Autodesk Inventor part; units mm, degrees
ref_plane "YZ Plane" through (0, 0, 0) normal (1, 0, 0) x (0, 1, 0)
ref_plane "XZ Plane" through (0, 0, 0) normal (0, 1, 0) x (-1, 0, 0)
ref_plane "XY Plane" through (0, 0, 0) normal (0, 0, 1) x (1, 0, 0)
sketch "Sketch1" plane through (0, 0, 0) normal (0, 1, 0) x (-1, 0, 0)
  line L0 (0, 0) -> (0, -86)
  line L1 (0, -86) -> (128.3, -86)
  line L2 (128.3, -86) -> (128.3, 0)
  line L3 (128.3, 0) -> (0, 0)
  dimension "d0" = 86
  dimension "d1" = 128.3
extrude "Extrusion2" add sketch "Sketch1" along normal blind 6
sketch "Sketch3" plane through (0, 6, 0) normal (0, 1, 0) x (1, 0, 0)
  point P0 (0, 0)
sketch "Sketch4" plane through (0, 6, 0) normal (0, 1, 0) x (1, 0, 0)
  arc A0 (-91.2531, 56.696) -> (-91.5743, 29.7143) centre (-95.2962, 43.2514) ccw
  arc A1 (-93.1804, 51.2354) -> (-93.1804, 34.2112) centre (-94.0166, 42.7233) ccw
  line L0 (-93.1804, 51.2354) -> (-91.2531, 56.696)
  line L1 (-93.1804, 34.2112) -> (-91.5743, 29.7143)
  arc A2 (-78.0632, 52.0407) -> (-78.3199, 34.448) centre (-76.5372, 43.2202) ccw
  arc A3 (-74.7545, 34.448) -> (-75.0113, 52.0407) centre (-76.5372, 43.2202) ccw
  arc A4 (-75.0113, 29.7143) -> (-75.0113, 56.696) centre (-76.1328, 43.2051) ccw
  line L2 (-75.0113, 56.696) -> (-75.0113, 52.0407)
  line L3 (-74.7545, 34.448) -> (-75.0113, 29.7143)
  line L4 (-78.3199, 34.448) -> (-78.3199, 29.4603)
  line L5 (-78.0632, 56.6961) -> (-78.0632, 52.0407)
  arc A5 (-78.0632, 56.6961) -> (-78.3199, 29.4603) centre (-77.9302, 43.0757) ccw
  line L6 (-59.5494, 56.6961) -> (-59.5494, 29.4603)
  line L7 (-59.5494, 29.4603) -> (-55.5494, 29.4603)
  line L8 (-55.5494, 29.4603) -> (-55.5494, 56.6961)
  line L9 (-55.5494, 56.6961) -> (-59.5494, 56.6961)
  line L10 (-47.4135, 29.4603) -> (-53.7861, 43.0782)
  arc A6 (-53.7861, 43.0782) -> (-53.7861, 54.3684) centre (-53.0876, 48.7233) ccw
  line L11 (-47.4135, 29.4603) -> (-43.9803, 31.0669)
  line L12 (-43.9803, 31.0669) -> (-48.5954, 40.9288)
  arc A7 (-48.5954, 40.9288) -> (-53.7861, 56.6961) centre (-52.5494, 48.3652) ccw
  line L13 (-53.7861, 56.6961) -> (-53.7861, 54.3684)
  line L14 (-41.5494, 56.0046) -> (-41.5494, 29.4603)
  line L15 (-41.5494, 29.4603) -> (-27.5494, 29.4603)
  line L16 (-27.5494, 29.4603) -> (-27.5494, 33.1666)
  line L17 (-27.5494, 33.1666) -> (-37.5494, 33.1666)
  line L18 (-37.5494, 33.1666) -> (-37.5494, 41.4179)
  line L19 (-37.5494, 41.4179) -> (-29.2175, 41.4179)
  line L20 (-29.2175, 41.4179) -> (-29.2175, 44.4179)
  line L21 (-29.2175, 44.4179) -> (-37.5494, 44.4179)
  line L22 (-37.5494, 44.4179) -> (-37.5494, 52.4179)
  line L23 (-37.5494, 52.4179) -> (-27.5494, 52.4179)
  line L24 (-27.5494, 52.4179) -> (-27.5494, 56.0046)
  line L25 (-27.5494, 56.0046) -> (-41.5494, 56.0046)
  line L26 (-128.3, 86) -> (-128.3, 0)
  line L27 (0, 86) -> (-128.3, 86)
  point P0 (0, 0)
extrude "Extrusion3" cut sketch "Sketch4" against normal through all
sketch "Sketch26" plane through (0, 6, 0) normal (0, 1, 0) x (1, 0, 0)
  point P0 (0, 0)
sketch "Sketch27" plane through (0, 6, 0) normal (0, 1, 0) x (1, 0, 0)
  line L0 (-1.7618, -2.4025) -> (1.922, -2.4025)
  point P0 (0, 0)
sketch "Sketch28" plane through (0, 6, 0) normal (0, 1, 0) x (1, 0, 0)
  point P0 (0, 0)
sketch "Sketch29" plane through (0, 6, 0) normal (0, 1, 0) x (1, 0, 0)
  line L0 (0, 86) -> (-128.3, 86)
  line L1 (-128.3, 86) -> (0, 86)
  line L2 (-128.3, 0) -> (0, 0)
  line L3 (0, 86) -> (0, 0)
  line L4 (0, 0) -> (-128.3, 0)
  line L5 (-128.3, 0) -> (-128.3, 86)
  line L6 (-137.3, -9) -> (-137.3, 95)
  line L7 (-137.3, 95) -> (9, 95)
  line L8 (9, 95) -> (9, -9)
  line L9 (9, -9) -> (-137.3, -9)
  dimension "d114" = 9
  dimension "d115" = 9
  dimension "d116" = 9
  dimension "d117" = 9
extrude "Extrusion11" add sketch "Sketch29" along normal blind 30 and the other way blind 6
sketch "Sketch30" plane through (-137.3, 36, 9) normal (0, 0, 1) x (1, 0, 0)
  line L0 (9, 0) -> (137.3, 0)
  arc A0 (53.4147, 0) -> (92.5853, 0) centre (73, -4.0519) ccw
  line L1 (53.4147, 0) -> (92.5853, 0)
  line L2 (0, -36) -> (0, 0)
  point P0 (137.3, -36)
  dimension "d160" = 20
  dimension "d161" = 73
extrude "Extrusion12" cut sketch "Sketch30" against normal through all
sketch "Sketch31" plane through (-137.3, 0, 9) normal (0, 0, 1) x (1, 0, 0)
  circle A0 centre (21.5643, 25) radius 3.25
  circle A1 centre (124.1286, 25) radius 3.25
  line L0 (146.3, 0) -> (0, 0)
  point P0 (137.3, 0)
  dimension "d124" = 6.5
  dimension "d125" = 6.5
  dimension "d126" = 25
  dimension "d127" = 25
extrude "Extrusion13" cut sketch "Sketch31" against normal through all
sketch "Sketch32" plane through (-128.3, 6, -86) normal (0, 0, 1) x (1, 0, 0)
  circle A0 centre (115.1286, 19) radius 3.25
  circle A1 centre (115.1286, 19) radius 5.25
  circle A2 centre (12.5643, 19) radius 3.25
  circle A3 centre (12.5643, 19) radius 5.25
  point P0 (128.3, -6)
  dimension "d130" = 10.5
  dimension "d131" = 10.5
extrude "Extrusion14" cut sketch "Sketch32" against normal blind 6.2
sketch "Sketch33" plane through (0, 6, 0) normal (0, 0, -1) x (-1, 0, 0)
  circle A0 centre (13.1714, 19) radius 3.25
  circle A1 centre (13.1714, 19) radius 5.25
  circle A2 centre (115.7357, 19) radius 3.25
  circle A3 centre (115.7357, 19) radius 5.25
  point P0 (0, -6)
  dimension "d134" = 10.5
  dimension "d135" = 10.5
extrude "Extrusion15" cut sketch "Sketch33" against normal blind 6.2
sketch "Sketch34" plane through (-137.3, 0, 9) normal (-1, 0, 0) x (0, 0, 1)
  line L0 (-9, 36) -> (-95, 36)
  line L1 (-104, 0) -> (-104, 36)
  arc A0 (-64.5, 36) -> (-39.5, 36) centre (-52, 34.966) ccw
  point P0 (-9, 0)
  dimension "d143" = 25
extrude "Extrusion16" cut sketch "Sketch34" against normal through all
sketch "Sketch35" plane through (-137.3, 0, -95) normal (-1, 0, 0) x (0, 0, 1)
  circle A0 centre (82, 25) radius 3.25
  circle A1 centre (22, 25) radius 3.25
  line L0 (104, 0) -> (0, 0)
  line L1 (0, 0) -> (0, 36)
  point P0 (95, 0)
  dimension "d144" = 6.5
  dimension "d145" = 6.5
  dimension "d146" = 25
  dimension "d147" = 25
  dimension "d150" = 60
  dimension "d151" = 22
extrude "Extrusion17" cut sketch "Sketch35" against normal through all
sketch "Sketch36" plane through (0, 6, -86) normal (-1, 0, 0) x (0, 0, 1)
  circle A0 centre (13, 19) radius 3.25
  circle A1 centre (13, 19) radius 5.25
  circle A2 centre (73.1913, 19) radius 5.25
  point P0 (86, -6)
  dimension "d152" = 10.5
  dimension "d153" = 10.5
extrude "Extrusion18" cut sketch "Sketch36" against normal blind 6.2 contours A0 | A1 | A2
sketch "Sketch37" plane through (-128.3, 6, 0) normal (1, 0, 0) x (0, 0, -1)
  circle A0 centre (13, 19) radius 3.25
  circle A1 centre (13, 19) radius 5.25
  circle A2 centre (73, 19) radius 3.25
  circle A3 centre (73, 19) radius 5.25
  point P0 (0, -6)
  dimension "d156" = 10.5
  dimension "d157" = 10.5
extrude "Extrusion19" cut sketch "Sketch37" against normal blind 6.2 contours A0 | A1 | A2 | A3
sketch "Sketch39" plane through (0, 0, 0) normal (0, -1, 0) x (1, 0, 0)
  line L0 (-84.3, 9) -> (-44.3, 9)
  line L1 (-64.3, 9) -> (-69.3, 9)
  line L2 (-69.3, 9) -> (-69.3, 12.3114)
  line L3 (-69.3, 12.3114) -> (-59.3, 12.3114)
  line L4 (-59.3, 12.3114) -> (-59.3, 9)
  arc A0 (-59.3, 12.3114) -> (-69.3, 12.3114) centre (-64.3, 17.2104) ccw
  line L5 (-64.3, -95.7654) -> (-69.3, -95.7654)
  line L6 (-69.3, -95.7654) -> (-69.3, -92.2822)
  line L7 (-69.3, -92.2822) -> (-59.3, -92.2822)
  line L8 (-59.3, -92.2822) -> (-59.3, -95.7654)
  arc A1 (-59.3, -92.2822) -> (-69.3, -92.2822) centre (-64.3, -87.3832) ccw
  line L9 (-59.3, -95.7654) -> (-64.3, -95.7654)
  line L10 (-44.3, -95) -> (-84.3, -95)
  point P0 (0, 0)
  point P1 (-44.7147, 9)
  point P2 (-83.8853, 9)
  point P3 (-83.8853, -95)
  point P4 (-44.7147, -95)
  point P5 (-69.3, -95)
  point P6 (-59.3, -95)
  dimension "d162" = 5
  dimension "d163" = 10
  dimension "d164" = 7
  dimension "d165" = 5
  dimension "d166" = 10
  dimension "d167" = 7
  dimension "d168" = 0
extrude "Extrusion20" cut sketch "Sketch39" against normal blind 20 contours L6 L7 L8 L10 | A1 L7
sketch "Sketch40" plane through (0, 0, 0) normal (0, -1, 0) x (1, 0, 0)
  line L0 (-84.2, 8.8958) -> (-44.2, 8.8958)
  line L1 (-64.2, 8.8958) -> (-69.2, 8.8958)
  line L2 (-69.2, 8.8958) -> (-69.2, 12.2072)
  line L3 (-69.2, 12.2072) -> (-59.2, 12.2072)
  line L4 (-59.2, 12.2072) -> (-59.2, 8.8958)
  arc A0 (-59.2, 12.2072) -> (-69.2, 12.2072) centre (-64.2, 17.1062) ccw
  line L5 (-64.2, -95.7654) -> (-69.3, -95.7654)
  line L6 (-69.3, -95.7654) -> (-69.3, -92.2822)
  line L7 (-69.3, -92.2822) -> (-59.1, -92.2822)
  line L8 (-59.1, -92.2822) -> (-59.1, -95.7654)
  arc A1 (-59.1, -92.2822) -> (-69.3, -92.2822) centre (-64.2, -86.7831) ccw
  line L9 (-59.1, -95.7654) -> (-64.2, -95.7654)
  line L10 (-44.3, -95) -> (-84.3, -95)
  point P0 (0, 0)
  point P1 (0, 0)
  point P2 (-44.7147, 9)
  point P3 (-83.8853, 9)
  point P4 (-44.2, 8.8958)
  point P5 (-83.8853, -95)
  point P6 (-44.7147, -95)
  point P7 (-69.3, -95)
  point P8 (-59.3, -95)
  dimension "d171" = 5
  dimension "d172" = 10
  dimension "d173" = 7
  dimension "d174" = 5.1
  dimension "d175" = 10.2
  dimension "d176" = 7.5
  dimension "d177" = 0
  dimension "d187" = 10.2
extrude "Extrusion21" add sketch "Sketch40" against normal blind 12 contours L2 L3 L4 L0 | A0 L3
chamfer "Chamfer1" distance 4 angle 45 2 edges at (9, 18, 9) (9, 18, -95)
chamfer "Chamfer2" distance 4 angle 45 2 edges at (-137.3, 18, 9) (-137.3, 18, -95)
properties part number "Rack holder aluminium"
Geometry check sheet. Reference: the model listing, model coordinates, mm. A direction names the side the tool comes from. Coordinates: 2 decimals unless noted, no trailing zeros. Loops run counter-clockwise (first coordinate to the right, second up) from the corner with the lowest first, then second, coordinate; pieces in that order, holes last. Notation, with made-up numbers: (-35.5, 51) - (7.5, 51) arc R36 ccw to (7.5, 89) - close; hole circle Ø8 at (-14.75, 74). An arc over 180 degrees is marked (long way). One line per item, written item: value. Start each with the question number.
(1) Cross-section at D-D on y = 25. Count the separate pieces of the cut face and the enclosed holes in it, plus the area to 3 significant figures.
(2) Mould release check, pull along Z, two halves, no side actions. Record for faces 1 (the cylindrical face through (-62.6, 3, -42.9)), 2 (the flat face through (-99, 21, -86)), 3 (the flat face through (-14, 36, 1)), 4 (the flat face through (7, 18, 7)): released by +Z, released by -Z, zero draft, split by the parting line, or undercut.
(3) Depth check by flat-ended pin: P1, Ø10.5, axis at y = 25, z = -13, coming from the +X side; P2, Ø6, axis at x = -83, y = 22, coming from the +Z side; P3, Ø12, axis at x = -46, z = -58.5, coming from the +Y side. Enter the tip coordinate at first touch or a pass-through.
(4) Material ranges on line 1 (Z direction, x = -21.5, y = 29); line 2 (X direction, y = 27, z = -82); line 3 (X direction, y = 21.5, z = 1), recorded low to high. Write a range as [from, to].
(5) Cross-section at C-C on z = -6. Enter the section's corners in (x, y).
(6) Tool access check on faces 5 (the flat face through (-16, 23, -92.2)), 6 (the flat face through (-45.721, 3.042, -30.252)). Record the directions out of +Z, -Z, +X, -X, +Y, -Y that give a thin tool (end or side, any length) a straight path to the whole face; none if there is none.
(7) Cross-section at A-A on z = -73. Enter the section's corners in (x, y), plus the area to 3 significant figures.
(8) Cross-section at B-B on y = 15.5. Enter the section's corners in (x, z).
Results below:
1. separate pieces: 12
1. enclosed holes: 0
1. area: 2,530 mm2
2. face 1: undercut
2. face 2: undercut
2. face 3: zero draft
2. face 4: released by +Z
3. P1: stops at x = 9
3. P2: stops at z = 9
3. P3: stops at y = 6
4. line 1: z = [-95, -86], [0, 9]
4. line 2: x = [-137.3, -128.3], [0, 9]
4. line 3: x = [-137.3, -119.65], [-111.82, -81.35], [-47.25, -17.08], [-9.26, 9]
5. outline: (-137.3, 0) - (9, 0) - (9, 36) - (0, 36) - (0, 6) - (-128.3, 6) - (-128.3, 36) - (-137.3, 36) - close
6. face 5: none
6. face 6: +Y, -Y
7. outline: (-137.3, 0) - (9, 0) - (9, 21.75) - (6.2, 21.75) - (6.2, 19.75) - (0, 19.75) - (0, 6) - (-128.3, 6) - (-128.3, 19.75) - (-134.5, 19.75) - (-134.5, 21.75) - (-137.3, 21.75) - close; (-137.3, 28.25) - (-134.5, 28.25) - (-134.5, 30.25) - (-128.3, 30.25) - (-128.3, 36) - (-137.3, 36) - close; (0, 30.25) - (6.2, 30.25) - (6.2, 28.25) - (9, 28.25) - (9, 36) - (0, 36) - close
7. area: 1,250 mm2
8. outline: (-137.3, -91) - (-133.3, -95) - (-75.68, -95) - (-75.68, -86) - (-128.3, -86) - (-128.3, 0) - (-75.68, 0) - (-75.68, 9) - (-133.3, 9) - (-137.3, 5) - close; (-52.92, -95) - (5, -95) - (9, -91) - (9, 5) - (5, 9) - (-52.92, 9) - (-52.92, 0) - (0, 0) - (0, -86) - (-52.92, -86) - close
